Can you work these out from the model? Positions are in its coordinate system, mm. Give positions to 0.01 mm unless a question says otherwise; leave off trailing zeros. Order: outer loops, then holes, each group sorted by start corner. A loop starts at its lowest first (then second) coordinate and runs counter-clockwise, first axis right, second up. Notation, with made-up numbers: M -5,63.5 L 13,63.5 A25 cw 13,81.5 Z; hole C 7.25,-9 d1. An arc over 180 degrees is marked long. Answer as a JSON object with one key per item and string values.
Autodesk Inventor part; units mm, degrees
ref_plane "MSC_PT1" through (0, 0, 2.2) normal (0, 0, 1) x (1, 0, 0)
ref_plane "MSC_PT2" through (0, 0, 0) normal (0, 0, -1) x (-1, 0, 0)
ref_plane "MSC_PF1" through (0, 0, 0) normal (1, 0, 0) x (0, 1, 0)
sketch "Sketch1" plane through (0, 0, 0) normal (0, 0, 1) x (1, 0, 0)
  circle A0 centre (0, 0) radius 3.5 construction
  line L0 (-3.5, 2.0207) -> (-3.5, -2.0207)
  line L1 (-3.5, -2.0207) -> (0, -4.0415)
  line L2 (0, -4.0415) -> (3.5, -2.0207)
  line L3 (3.5, -2.0207) -> (3.5, 2.0207)
  line L4 (3.5, 2.0207) -> (0, 4.0415)
  line L5 (0, 4.0415) -> (-3.5, 2.0207)
  line L6 (0, 5.658) -> (0, -5.658)
  line L7 (-4.9, 0) -> (4.9, 0)
  point P0 (0, 0)
  dimension "ParS" = 7
extrude "Extrusion1" add sketch "Sketch1" along normal blind 2.2
sketch "Sketch2" plane through (0, 0, 2.2) normal (0, 0, 1) x (1, 0, 0)
  point P0 (0, 0)
  point P1 (0, 0)
hole "Hole1" at (0, 0, 2.2) direction (0, 0, -1) diameter 3.242 end through all
ref_plane "MSC_PT1" through (0, 0, 2.2) normal (0, 0, 1) x (1, 0, 0)
ref_plane "MSC_PT2" through (0, 0, 0) normal (0, 0, -1) x (-1, 0, 0)
ref_plane "MSC_PF1" through (0, 0, 0) normal (1, 0, 0) x (0, 1, 0)
chamfer "Chamfer1" distance 0.42 angle 45 2 edges at (0, 1.621, 2.2) (0, 1.621, 0)
equation "\"d17\" = 0.6 * PTC"
equation "\"d18\" = 0.6 * PTC"
equation "\"d4\" = M"
equation "\"PTC\" = 0.7"
equation "\"NND\" = 4"
equation "\"THREADDIA\" = NND"
properties part number "ISO 4036 - M4" material "Steel"
1) I want a section at B-B on z = 1.55. Write out the boundary of the cut face in (x, y).
Results found:
{"outline": "M -3.5,-2.02 L 0,-4.04 L 3.5,-2.02 L 3.5,2.02 L 0,4.04 L -3.5,2.02 Z; hole C 0,0 d3.24"}
2) I want a section at C-C on y = 2.25. Write out the boundary of the cut face in (x, z), and give its area (3 significant figures).
Results found:
{"outline": "M -3.1,0 L 3.1,0 L 3.1,2.2 L -3.1,2.2 Z", "area": "13.7 mm²"}
3) I want a section at A-A on y = 0. Write out the boundary of the cut face in (x, z).
Results found:
{"outline": "M -3.5,0 L -2.04,0 L -1.62,0.42 L -1.62,1.78 L -2.04,2.2 L -3.5,2.2 Z; M 1.62,0.42 L 2.04,0 L 3.5,0 L 3.5,2.2 L 2.04,2.2 L 1.62,1.78 Z"}
4) Thinking about a two-plate mould opening in Y: for faces 1 (the face through (1.8, 3, 1.1)), 2 (the face through (-2, -2, 0)), 3 (the face through (1.438, -0.748, 1.09)), 4 (the face through (1.726, -3.045, 1.085)), which applies, pulls with the +Y half, pulls with the -Y half, needs draft (parallel to the pull), parting line crosses it, or undercut?
Results found:
{"face 1": "pulls with the +Y half", "face 2": "needs draft", "face 3": "undercut", "face 4": "pulls with the -Y half"}
5) I need wall thicknesses on L1, parallel to X at y = 0, z = 1.1; L2, parallel to Y at x = 0.25, z = 1; L3, parallel to Y at x = 0.75, z = 0.55. Which ranges of each line are inside material? Lowest first, please.
Results found:
{"L1": "x = -3.5 to -1.62, 1.62 to 3.5", "L2": "y = -3.9 to -1.6, 1.6 to 3.9", "L3": "y = -3.61 to -1.44, 1.44 to 3.61"}
